```python
from build123d import *

# Parameters (mm, degrees)
F1_DEPTH  = 25
F2_R      = 1.55
F3_DEPTH  = 25
F4_R      = 1.5
F5_DEPTH  = 25
F6_R      = 3.3134143982
F9_DEPTH  = 1.2
F8_R      = 1.5
F10_DEPTH = 1.2
F12_DEPTH = 1.2
F13_R     = 0.5


# Not quite as in the source:
# - ends of sketch curves that miss each other by under 0.0002 mm in the source are joined


with BuildPart() as f1:
    # F0 (on Front) → F1 (new body)
    with BuildSketch(Plane.XZ):
        with BuildLine():
            Line((-30, -27.2712218283), (30, -27.271222222))
            Line((30, -27.271222222), (30, -22.271222222))
            Line((30, -22.271222222), (12.3570600307, -22.2712218283))
            ThreePointArc((12.3570600307, -22.2712218283), (16.8965495982, -8.7237267257), (9.5007861894, 3.5010134632))
            Line((9.5007861894, 3.5010134632), (9.5007861894, 13.5010134632))
            Line((9.5007861894, 13.5010134632), (3, 13.5010134632))
            Line((3, 13.5010134632), (3, 6.1368714524))
            Line((3, 6.1368714524), (3, 4.8868714524))
            Line((3, 4.8868714524), (3, 1.0226200218))
            ThreePointArc((3, 1.0226200218), (0, -22.5963300169), (-3, 1.0226200218))
            Line((-3, 1.0226200218), (-3, 4.8868714524))
            Line((-3, 4.8868714524), (-3, 13.5010134632))
            Line((-3, 13.5010134632), (-9.5007861894, 13.5010134632))
            Line((-9.5007861894, 13.5010134632), (-9.5007861894, 3.5010134632))
            ThreePointArc((-9.5007861894, 3.5010134632), (-16.8965495982, -8.7237267257), (-12.3570600307, -22.2712218283))
            Line((-12.3570600307, -22.2712218283), (-30, -22.2712218283))
            Line((-30, -22.2712218283), (-30, -27.2712218283))
        make_face()
    extrude(amount=F1_DEPTH)

    # F2 (on face) → F3 (cut)
    with BuildSketch(Plane.XY.offset(-22.2712218283)):
        with Locations((-25, -12.5)):
            Circle(F2_R)
        with Locations((25, -12.5)):
            Circle(F2_R)
    extrude(amount=-F3_DEPTH, mode=Mode.SUBTRACT)

    # F4 (on face) → F5 (cut)
    with BuildSketch(Plane.YZ.offset(9.5007861894)):
        with Locations((-18.75, 8.5010134632)):
            Circle(F4_R)
        with Locations((-6.25, 8.5010134632)):
            Circle(F4_R)
    extrude(amount=-F5_DEPTH, mode=Mode.SUBTRACT)

    # F6
    f6_edges = [f1.edges().sort_by_distance(p)[0] for p in [
        (-6.250393, -25, 13.501013),
        (6.250393, -25, 13.501013),
        (-6.250393, 0, 13.501013),
        (6.250393, 0, 13.501013),
        (30, -25, -24.771222),
        (30, 0, -24.771222),
        (-30, 0, -24.771222),
        (-30, -25, -24.771222),
        (12.35706, -12.5, -22.271222),
        (-12.35706, -12.5, -22.271222),
    ]]
    fillet(f6_edges, radius=F6_R)

    # F7 (on face) → F9 (cut)
    with BuildSketch(Plane.YZ.offset(9.5007861894)):
        Polygon((-20.55, 5.3833220096), (-16.95, 5.3833220096), (-15.15, 8.5010134632), (-16.95, 11.6187049168), (-20.55, 11.6187049168), (-22.35, 8.5010134632), align=None)
        Polygon((-4.45, 11.6187049168), (-8.05, 11.6187049168), (-9.85, 8.5010134632), (-8.05, 5.3833220096), (-4.45, 5.3833220096), (-2.65, 8.5010134632), align=None)
    extrude(amount=-F9_DEPTH, mode=Mode.SUBTRACT)

    # F8 (on face) → F10 (cut)
    with BuildSketch(Plane(origin=(-9.5007861894, 0, 0), x_dir=(0, -1, 0), z_dir=(-1, 0, 0))):
        Polygon((4.45, 5.3833220096), (8.05, 5.3833220096), (9.85, 8.5010134632), (8.05, 11.6187049168), (4.45, 11.6187049168), (2.65, 8.5010134632), align=None)
        with Locations((6.25, 8.5010134632)):
            Circle(F8_R, mode=Mode.SUBTRACT)
        Polygon((20.55, 11.6187049168), (16.95, 11.6187049168), (15.15, 8.5010134632), (16.95, 5.3833220096), (20.55, 5.3833220096), (22.35, 8.5010134632), align=None)
        with Locations((18.75, 8.5010134632)):
            Circle(F8_R, mode=Mode.SUBTRACT)
    extrude(amount=-F10_DEPTH, mode=Mode.SUBTRACT)

    # F11 (on face) → F12 (cut)
    with BuildSketch(Plane.XY.offset(-22.2712218283)):
        Polygon((26.8, -9.3823085464), (23.2, -9.3823085464), (21.4, -12.5), (23.2, -15.6176914536), (26.8, -15.6176914536), (28.6, -12.5), align=None)
        Polygon((-23.2, -15.6176914536), (-21.4, -12.5), (-23.2, -9.3823085464), (-26.8, -9.3823085464), (-28.6, -12.5), (-26.8, -15.6176914536), align=None)
    extrude(amount=-F12_DEPTH, mode=Mode.SUBTRACT)

    # F13
    f13_edges = [f1.edges().sort_by_distance(p)[0] for p in [
        (0, 0, -22.59633),
        (0, -25, -22.59633),
    ]]
    fillet(f13_edges, radius=F13_R)


solid = f1.part
```
Model file for the job. Use its own axes, mm. A direction names the side the tool comes from. Give positions to 0.01 mm unless a question says otherwise; leave off trailing zeros. Loops run counter-clockwise (first coordinate to the right, second up) from the corner with the lowest first, then second, coordinate; pieces in that order, holes last. Notation, with made-up numbers: (81, 23) -> (133, 23) arc R33 ccw to (133, 51) -> close; hole circle Ø11 at (-4, 42). An arc over 180 degrees is marked (long way). Write each question's results on one line, items separated by ' | '.
(1) Cut at A-A on y = -11.75. Give the number of separate pieces and of enclosed holes in the cut face, and give its area (3 significant figures).
Geometry results:
separate pieces: 3 | enclosed holes: 0 | area: 723 mm²
(2) Cut at C-C on x = 0. List the corners of the cut face in (y, z).
Geometry results:
outline: (-25, -27.27) -> (0, -27.27) -> (0, -23.1) arc R0.5 ccw to (-0.5, -22.6) -> (-24.5, -22.6) arc R0.5 ccw to (-25, -23.1) -> close
(3) Tool access for faces 4 (the flat face through (-9, -6, 5.383)), 5 (the cylindrical face through (5.69, -7.36, 9.51)), 6 (the flat face through (8.909, -3.563, 6.92)), 7 (the flat face through (27.69, -14.08, -22.86)): list every direction of +Z, -Z, +X, -X, +Y, -Y with a clear straight run to the whole face (end or side of a thin tool).
Geometry results:
face 4: -X | face 5: +X, -X | face 6: +X | face 7: +Z
(4) Probe line 1 along X through (y, z) = (-1.25, 11); line 2 along Z through (x, y) = (-4.4, -6.25); line 3 along Z through (x, y) = (7.2, -18.75). List the from-to ranges inside material, lowest first.
Geometry results:
line 1: x = -9.5 to -3, 3 to 9.5 | line 2: z = -27.27 to -21.76, 0.57 to 7, 10 to 13.5 | line 3: z = -27.27 to -20.2, -1 to 7, 10 to 13.5
(5) Pull direction X, two halves, no side cores. Call faces 1 (the cylindrical face through (15.75, -12.68, -20.79)), 2 (the flat face through (-6, -12, 13.501)), 3 (the cylindrical face through (-25.336, -14.013, -25.345)): released by +X, released by -X, zero draft, split by the parting line, or undercut.
Geometry results:
face 1: released by +X | face 2: zero draft | face 3: undercut
(6) Cut at B-B on x = 25. List the corners of the cut face in (y, z).
Geometry results:
outline: (-25, -27.27) -> (-14.05, -27.27) -> (-14.05, -23.47) -> (-15.62, -23.47) -> (-15.62, -22.27) -> (-25, -22.27) -> close; (-10.95, -27.27) -> (0, -27.27) -> (0, -22.27) -> (-9.38, -22.27) -> (-9.38, -23.47) -> (-10.95, -23.47) -> close
(7) Flat gauge pins, fed straight in: pin 1 Ø3.5 at (x, y) = (-25, -12.5) entering from +Z; pin 2 Ø5 at (y, z) = (-5.5, 9) entering from -X; pin 3 Ø13.5 at (y, z) = (-12, 9.5) entering from +X. Where does each tip first touch, or does it go through?
Geometry results:
pin 1: stops at z = -23.47 | pin 2: stops at x = -9.5 | pin 3: stops at x = 10.53
